```python
from build123d import *

# Parameters (mm, degrees)
SKETCH1_W    = 425
SKETCH1_H    = 410
BOTTOM_DEPTH = 3.175
SKETCH2_W    = 425
SKETCH2_H    = 410
SKETCH2_W_2  = 420.428
SKETCH2_H_2  = 405.428
SKETCH2_W_3  = 2.286
SKETCH2_H_3  = 201.571
SKETCH2_W_4  = 209.071
SKETCH2_H_4  = 2.286
SIDES_DEPTH  = 246.6
SKETCH3_W    = 425
SKETCH3_H    = 410
TOP_DEPTH    = 2.286


with BuildPart() as part:
    # Sketch1 → Bottom (new body)
    with BuildSketch(Plane(origin=(0, 0, 0), x_dir=(1, 0, 0), z_dir=(0, 1, 0))):
        Rectangle(SKETCH1_W, SKETCH1_H)
    extrude(amount=BOTTOM_DEPTH)

    # Sketch2 → Sides (add)
    with BuildSketch(Plane(origin=(0, 3.175, 0), x_dir=(1, 0, 0), z_dir=(0, 1, 0))):
        Rectangle(SKETCH2_W, SKETCH2_H)
        Rectangle(SKETCH2_W_2, SKETCH2_H_2, mode=Mode.SUBTRACT)
        with Locations((0, 101.9285)):
            Rectangle(SKETCH2_W_3, SKETCH2_H_3)
        with Locations((105.6785, 0)):
            Rectangle(SKETCH2_W_4, SKETCH2_H_4)
        with Locations((0, -101.9285)):
            Rectangle(SKETCH2_W_3, SKETCH2_H_3)
        Rectangle(SKETCH2_W_3, SKETCH2_H_4)
        with Locations((-105.6785, 0)):
            Rectangle(SKETCH2_W_4, SKETCH2_H_4)
    extrude(amount=SIDES_DEPTH)

    # Sketch3 → Top (add)
    with BuildSketch(Plane(origin=(0, 249.775, 0), x_dir=(1, 0, 0), z_dir=(0, 1, 0))):
        Rectangle(SKETCH3_W, SKETCH3_H)
    extrude(amount=TOP_DEPTH)


solid = part.part
```
Source: CAD feature listing. Evaluate the final solid. Frame: model axes, mm. Round coordinates to 2 decimals unless told otherwise and drop trailing zeros. Loops run counter-clockwise (first coordinate to the right, second up) from the corner with the lowest first, then second, coordinate; pieces in that order, holes last. Notation, with made-up numbers: M -5,22.5 L 31,22.5 A20 cw 31,39.5 Z; hole C -3,18.25 d3. An arc over 180 degrees is marked long. Put each result on its own line as item: value.
(1) Section A-A, the plane x = -61.5. Return loops of the section in (y, z) (3 decimals).
Solutions:
outline: M 0,-205 L 252.061,-205 L 252.061,205 L 0,205 Z; hole M 3.175,-202.714 L 249.775,-202.714 L 249.775,-1.143 L 3.175,-1.143 Z; hole M 3.175,1.143 L 249.775,1.143 L 249.775,202.714 L 3.175,202.714 Z
(2) Ray query, line 1 (Z direction, x = 126, y = 18); line 2 (X direction, y = 99.5, z = -45.5); line 3 (Y direction, x = 189.5, z = 120.5) (3 decimals). Return the intervals inside material, ascending. Write a range as [from, to].
Solutions:
line 1: [-205, -202.71], [-1.14, 1.14], [202.71, 205]
line 2: [-212.5, -210.21], [-1.14, 1.14], [210.21, 212.5]
line 3: [0, 3.175], [249.775, 252.061]
(3) Section B-B, the plane z = 149. Return loops of the section in (x, y) (3 decimals), and give its area (3 significant figures).
Solutions:
outline: M -212.5,0 L 212.5,0 L 212.5,252.061 L -212.5,252.061 Z; hole M -210.214,3.175 L -1.143,3.175 L -1.143,249.775 L -210.214,249.775 Z; hole M 1.143,3.175 L 210.214,3.175 L 210.214,249.775 L 1.143,249.775 Z
area: 4,010 mm²
(4) Section C-C, the plane y = 225.5. Return loops of the section in (x, z).
Solutions:
outline: M -212.5,-205 L 212.5,-205 L 212.5,205 L -212.5,205 Z; hole M -210.21,-202.71 L -1.14,-202.71 L -1.14,-1.14 L -210.21,-1.14 Z; hole M -210.21,1.14 L -1.14,1.14 L -1.14,202.71 L -210.21,202.71 Z; hole M 1.14,-202.71 L 210.21,-202.71 L 210.21,-1.14 L 1.14,-1.14 Z; hole M 1.14,1.14 L 210.21,1.14 L 210.21,202.71 L 1.14,202.71 Z
(5) Pull-direction query (Y, two-part tool) for faces 1 (the face through (-3, 124, -205)), 2 (the face through (-210.214, 125, 103)), 3 (the face through (-3, 0, -3)); classes: released by +Y, released by -Y, zero draft, split by the parting line, or undercut.
Solutions:
face 1: zero draft
face 2: undercut
face 3: released by -Y
